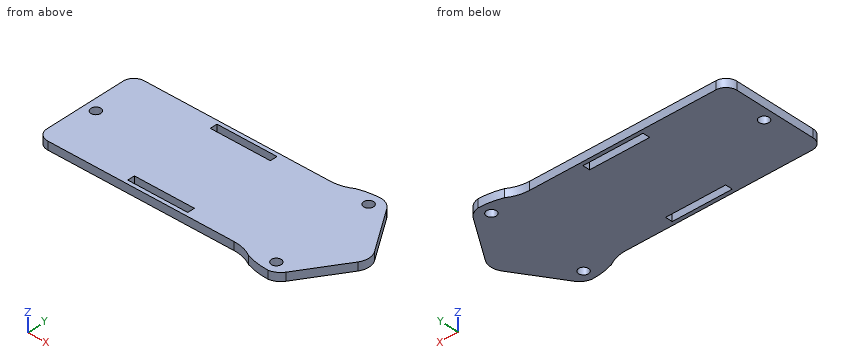
```python
from build123d import *

# Parameters (mm, degrees)
F0_W     = 22
F0_H     = 2.627969
F0_R     = 1.8
F1_DEPTH = 3


with BuildPart() as f1:
    # F0 (on Top) → F1 (new body)
    with BuildSketch(Plane.XY):
        with BuildLine():
            Line((-70.846429, 19), (-101.2, 19))
            ThreePointArc((-101.2, 19), (-104.028427, 17.828427), (-105.2, 15))
            Line((-105.2, 15), (-105.2, -15))
            ThreePointArc((-105.2, -15), (-104.028427, -17.828427), (-101.2, -19))
            Line((-101.2, -19), (-70.846429, -19))
            Line((-70.846429, -19), (-32.929577, -19))
            ThreePointArc((-32.929577, -19), (-29.172307, -19.531094), (-25.709437, -21.082761))
            ThreePointArc((-25.709437, -21.082761), (-21.550048, -22.143225), (-17.272454, -22.5))
            ThreePointArc((-17.272454, -22.5), (-14.912775, -21.629956), (-13.117664, -19.868527))
            Line((-13.117664, -19.868527), (-2.182587, -3.305832))
            ThreePointArc((-2.182587, -3.305832), (-1.18973, 0), (-2.182587, 3.305832))
            Line((-2.182587, 3.305832), (-13.117664, 19.868527))
            ThreePointArc((-13.117664, 19.868527), (-14.912775, 21.629956), (-17.272454, 22.5))
            ThreePointArc((-17.272454, 22.5), (-21.550048, 22.143225), (-25.709437, 21.082761))
            ThreePointArc((-25.709437, 21.082761), (-29.172307, 19.531094), (-32.929577, 19))
            Line((-32.929577, 19), (-70.846429, 19))
        make_face()
        with Locations((-62.2, -16.299169)):
            Rectangle(F0_W, F0_H, mode=Mode.SUBTRACT)
        with Locations((-18.2, -18.2)):
            Circle(F0_R, mode=Mode.SUBTRACT)
        with Locations((-101.2, 0)):
            Circle(F0_R, mode=Mode.SUBTRACT)
        with Locations((-62.2, 16.299169)):
            Rectangle(F0_W, F0_H, mode=Mode.SUBTRACT)
        with Locations((-18.2, 18.2)):
            Circle(F0_R, mode=Mode.SUBTRACT)
    extrude(amount=F1_DEPTH)


solid = f1.part
```
Can you work these out from the model? Positions are in its coordinate system, mm. Round coordinates to 2 decimals unless told otherwise and drop trailing zeros. Loops run counter-clockwise (first coordinate to the right, second up) from the corner with the lowest first, then second, coordinate; pieces in that order, holes last. Notation, with made-up numbers: M -19.5,29.5 L 31.5,29.5 A25 cw 31.5,47.5 Z; hole C 62.5,74 d10. An arc over 180 degrees is marked long. Write item = value, one per line. Start each with the question number.
(1) Suppose I cut it at B-B on y = 0. Write out the boundary of the cut face in (x, z).
(2) Suppose I cut it at D-D on x = -18.2. Write out the boundary of the cut face in (y, z).
(3) I need wall thicknesses on line 1 along Y through (x, z) = (-18.2, 1.2); line 2 along Y through (x, z) = (-66.5, 1.15); line 3 along Y through (x, z) = (-91.5, 1.1). Which ranges of each line are inside material? Lowest first, please.
(4) Suppose I cut it at C-C on z = 2.25. Write out the boundary of the cut face in (x, y), plus the area to 3 significant figures.
(5) Suppose I cut it at A-A on x = -63.5. Write out the boundary of the cut face in (y, z), plus the area to 3 significant figures.
(6) I'm going to push flat-ended pins straight in: P1, Ø1, axis at x = -51, z = 2.5, coming from the +Y side; P2, Ø3, axis at x = -18.2, y = 18.2, coming from the -Z side; P3, Ø0.9, axis at x = -62, z = 1.5, coming from the -Y side; P4, Ø0.8, axis at y = -16, z = 2, coming from the +X side. Where does each tip first touch, or does it pass through?
Answer block:
q1.outline = M -105.2,0 L -103,0 L -103,3 L -105.2,3 Z; M -99.4,0 L -1.19,0 L -1.19,3 L -99.4,3 Z
q2.outline = M -22.48,0 L -20,0 L -20,3 L -22.48,3 Z; M -16.4,0 L 16.4,0 L 16.4,3 L -16.4,3 Z; M 20,0 L 22.48,0 L 22.48,3 L 20,3 Z
q3.line_1 = -22.48 to -20, -16.4 to 16.4, 20 to 22.48
q3.line_2 = -19 to -17.61, -14.99 to 14.99, 17.61 to 19
q3.line_3 = -19 to 19
q4.outline = M -105.2,-15 A4 ccw -101.2,-19 L -32.93,-19 A13.56 cw -25.71,-21.08 A25.82 ccw -17.27,-22.5 A5.99 ccw -13.12,-19.87 L -2.18,-3.31 A6 ccw -2.18,3.31 L -13.12,19.87 A5.99 ccw -17.27,22.5 A25.82 ccw -25.71,21.08 A13.56 cw -32.93,19 L -101.2,19 A4 ccw -105.2,15 Z; hole C -101.2,0 d3.6; hole M -73.2,-17.61 L -51.2,-17.61 L -51.2,-14.99 L -73.2,-14.99 Z; hole M -73.2,14.99 L -51.2,14.99 L -51.2,17.61 L -73.2,17.61 Z; hole C -18.2,-18.2 d3.6; hole C -18.2,18.2 d3.6
q4.area = 3,690 mm²
q5.outline = M -19,0 L -17.61,0 L -17.61,3 L -19,3 Z; M -14.99,0 L 14.99,0 L 14.99,3 L -14.99,3 Z; M 17.61,0 L 19,0 L 19,3 L 17.61,3 Z
q5.area = 98.2 mm²
q6.P1 = 19
q6.P2 = through
q6.P3 = -19
q6.P4 = -10.3
